Geometry: final body of the model. Coordinates: model frame, mm. Face numbers are marked on the shaded views. A direction names the side the tool comes from. Give positions to 0.01 mm unless a question says otherwise; leave off trailing zeros. Loops run counter-clockwise (first coordinate to the right, second up) from the corner with the lowest first, then second, coordinate; pieces in that order, holes last. Notation, with made-up numbers: (55, 54.25) - (64, 54.25) arc R31 ccw to (64, 85.25) - close; hole circle Ø6 at (-24.5, 53.25). An arc over 180 degrees is marked (long way). Use one line per item in the form item = value.
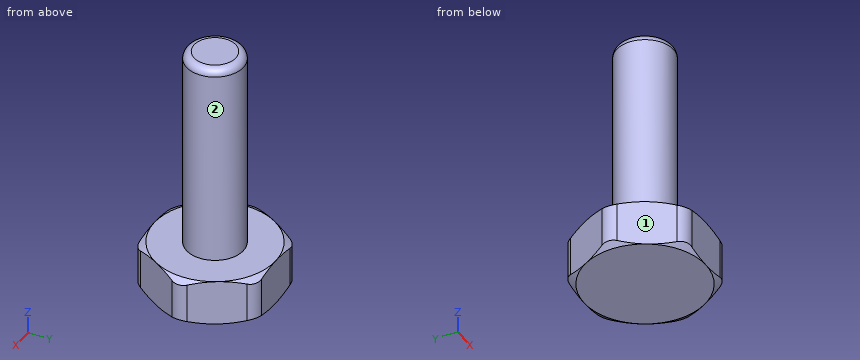
```python
from build123d import *

# Parameters (mm, degrees)
SKETCH4_R               = 1.875
BOSS_EXTRUDE2_DEPTH     = 1.5
SKETCH5_OUTSIDE_W       = 65.716
SKETCH5_OUTSIDE_H       = 64.478
SKETCH5_OUTSIDE_R       = 4
CUT_EXTRUDE1_DEPTH      = 15
CUT_EXTRUDE1_DRAFT      = -60
MIRROR1_COPY_1_SKETCH_W = 65.716
MIRROR1_COPY_1_SKETCH_H = 64.478
MIRROR1_COPY_1_SKETCH_R = 4
MIRROR1_COPY_1_DEPTH    = 15
MIRROR1_COPY_1_DRAFT    = -60
SKETCH4_3_R             = 1.875
BOSS_EXTRUDE3_DEPTH     = 15
FILLET1_R               = 1
FILLET2_R               = 0.5


with BuildPart() as part:
    # Sketch4 → Boss-Extrude2 (new, symmetric)
    with BuildSketch(Plane.XY):
        Polygon((4.618802154, 0), (2.309401077, 4), (-2.309401077, 4), (-4.618802154, 0), (-2.309401077, -4), (2.309401077, -4), align=None)
        Circle(SKETCH4_R, mode=Mode.SUBTRACT)
        Circle(SKETCH4_R)
    extrude(amount=BOSS_EXTRUDE2_DEPTH, both=True)


with BuildPart() as cut_extrude1_tool:
    # Sketch5 outside → Cut-Extrude1 (with draft: the straight prism first)
    with BuildSketch(Plane.XY.offset(1.5)):
        Rectangle(SKETCH5_OUTSIDE_W, SKETCH5_OUTSIDE_H)
        Circle(SKETCH5_OUTSIDE_R, mode=Mode.SUBTRACT)
    extrude(amount=-CUT_EXTRUDE1_DEPTH)
    # Cut-Extrude1: the draft: its side faces are tilted about the plane it starts from
    cut_extrude1_sides = [cut_extrude1_tool.faces().sort_by_distance(p)[0] for p in [
        (0, -32.239, -6),
        (32.858, 0, -6),
        (0, 32.239, -6),
        (-32.858, 0, -6),
        (-4, 0, -6),
    ]]
    draft(cut_extrude1_sides, Plane.XY.offset(1.5), CUT_EXTRUDE1_DRAFT)


with BuildPart() as part_1:
    add(part.part)

    # Cut-Extrude1: cut by cut_extrude1_tool
    add(cut_extrude1_tool.part, mode=Mode.SUBTRACT)


with BuildPart() as mirror1_copy_1_tool:
    # Mirror1 copy 1 sketch → Mirror1 copy 1 (with draft: the straight prism first)
    with BuildSketch(Plane(origin=(0, 0, -1.5), x_dir=(1, 0, 0), z_dir=(0, 0, -1))):
        Rectangle(MIRROR1_COPY_1_SKETCH_W, MIRROR1_COPY_1_SKETCH_H)
        Circle(MIRROR1_COPY_1_SKETCH_R, mode=Mode.SUBTRACT)
    extrude(amount=-MIRROR1_COPY_1_DEPTH)
    # Mirror1 copy 1: the draft: its side faces are tilted about the plane it starts from
    mirror1_copy_1_sides = [mirror1_copy_1_tool.faces().sort_by_distance(p)[0] for p in [
        (0, -32.239, 6),
        (32.858, 0, 6),
        (0, 32.239, 6),
        (-32.858, 0, 6),
        (-4, 0, 6),
    ]]
    draft(mirror1_copy_1_sides, Plane(origin=(0, 0, -1.5), x_dir=(1, 0, 0), z_dir=(0, 0, -1)), MIRROR1_COPY_1_DRAFT)


with BuildPart() as part_2:
    add(part_1.part)

    # Mirror1 copy 1: cut by mirror1_copy_1_tool
    add(mirror1_copy_1_tool.part, mode=Mode.SUBTRACT)

    # Sketch4_3 → Boss-Extrude3 (add)
    with BuildSketch(Plane.XY):
        Circle(SKETCH4_3_R)
    extrude(amount=BOSS_EXTRUDE3_DEPTH)

    # Fillet1
    fillet1_edges = [part_2.edges().sort_by_distance(p)[0] for p in [
        (4.618802154, 0, 0),
        (2.309401077, -4, 0),
        (-2.309401077, -4, 0),
        (-4.618802154, 0, 0),
        (-2.309401077, 4, 0),
        (2.309401077, 4, 0),
    ]]
    fillet(fillet1_edges, radius=FILLET1_R)

    # Fillet2
    fillet2_edges = [part_2.edges().sort_by_distance(p)[0] for p in [
        (-1.875, 0, 15),
    ]]
    fillet(fillet2_edges, radius=FILLET2_R)


solid = part_2.part
```
(1) Cut plane B-B (z = 10.75). Return the cut outline in (x, y) (3 decimals), plus the area to 3 significant figures.
Solution:
outline = circle Ø3.75 at (0, 0)
area = 11.0 mm2
(2) Pin query (flat end, axial travel): P1, Ø5, axis at x = -1.5, z = 6.5, coming from the -Y side (3 decimals); P2, Ø5, axis at x = -3, z = 8, coming from the +Y side; P3, Ø1.5, axis at x = 3.5, y = 3, coming from the +Z side. Return the tip coordinate at first contact, or that it passes through.
Solution:
P1 = -1.875
P2 = 1.81
P3 = 1.5
(3) Material intervals for L1, parallel to Z at x = -3.5, y = -1; L2, parallel to X at y = 0, z = 13 (3 decimals); L3, parallel to X at y = -3.5, z = 0, sorted ascending. Write a range as from..to.
Solution:
L1 = -1.5..1.5
L2 = -1.875..1.875
L3 = -2.6..2.6
(4) Access query for the marked faces 1 and 2. Directions: +Z, -Z, +X, -X, +Y, -Y. A direction counts if a zero-diameter tool reaches every point of the face in a straight line with its end or side. Return the directions, or none.
Solution:
face_1 = +Z, -Z, -X, -Y
face_2 = +Z
(5) Cut plane A-A (y = 0). Return the cut outline in (x, z) (3 decimals), plus the area to 3 significant figures.
Solution:
outline = (-4.464, -1.232) - (-4, -1.5) - (4, -1.5) - (4.464, -1.232) - (4.464, 1.232) - (4, 1.5) - (1.875, 1.5) - (1.875, 14.5) arc R0.5 ccw to (1.375, 15) - (-1.375, 15) arc R0.5 ccw to (-1.875, 14.5) - (-1.875, 1.5) - (-4, 1.5) - (-4.464, 1.232) - close
area = 77.1 mm2
